Can you work these out from the model? Positions are in its coordinate system, mm. A direction names the side the tool comes from. Round coordinates to 2 decimals unless told otherwise and drop trailing zeros. Order: outer loops, then holes, each group sorted by start corner. A loop starts at its lowest first (then second) coordinate and runs counter-clockwise, first axis right, second up.
Q1. If we section it at B-B (y = 37): Please give me the cut outline in (x, z), plus the area to 3 significant figures.
Q2. We'd pull the mould along Z, two halves only. Please class faces 1 (the face through (7, 0, -5)), 2 (the face through (6.8, 22.5, -4.7)), 3 (the face through (6.84, 44.4, -10.93)), 4 (the face through (7, 23, 0)): pulls with the +Z half, pulls with the -Z half, needs draft (parallel to the pull), parting line crosses it, or undercut.
Q3. For faces 5 (the face through (7, 45, -5)), 6 (the face through (7, 33, -8.681)), which set-ups out of +Z, -Z, +X, -X, +Y, -Y let a thin tool reach every point of the face, with its end or its side?
Q4. If we section it at C-C (z = -5.5): Please give me the cut outline in (x, y).
Q5. If we section it at A-A (z = -7.5): Please give me the cut outline in (x, y).
Q6. If I drill on line 1 (Z direction, x = 5.25, y = 43); line 2 (Y direction, x = 5.25, z = -6.5); line 3 (Y direction, x = 8.5, z = -5.5), over which ranges is the centre line in solid material (lowest first)?
Q7. If we section it at D-D (x = 7.25): Please give me the cut outline in (y, z).
Autodesk Inventor part; units mm, degrees
ref_plane "YZ Plane" through (0, 0, 0) normal (1, 0, 0) x (0, 1, 0)
ref_plane "XZ Plane" through (0, 0, 0) normal (0, 1, 0) x (-1, 0, 0)
ref_plane "XY Plane" through (0, 0, 0) normal (0, 0, 1) x (1, 0, 0)
sketch "スケッチ1" plane through (0, 0, 0) normal (1, 0, 0) x (0, 1, 0)
  line L0 (45, 0) -> (0, 0)
  line L1 (0, 0) -> (0, -11.5)
  line L2 (0, -11.5) -> (45, -11.5)
  line L3 (45, -11.5) -> (45, 0)
  dimension "d0" = 45
  dimension "d1" = 11.5
extrude "押し出し1" add sketch "スケッチ1" along normal blind 13.5
sketch "スケッチ2" plane through (13.5, 0, 0) normal (1, 0, 0) x (0, 0, -1)
  circle A0 centre (1.5, 43) radius 0.8
  circle A1 centre (9.4807, 43) radius 0.8
  circle A2 centre (9.5, 2) radius 0.8
  circle A3 centre (1.5, 2) radius 0.8
  circle A4 centre (5.5, 22.5) radius 0.8
  point P0 (0, 0)
extrude "押し出し2" cut sketch "スケッチ2" against normal through all
fillet "フィレット1" radius 2 2 edges at (6.75, 45, -11.5) (6.75, 0, -11.5)
sketch "スケッチ4" plane through (13.5, 0, 0) normal (1, 0, 0) x (0, 0, -1)
  line L0 (2.3, 40) -> (8.6807, 40)
  line L1 (8.6807, 40) -> (8.6807, 25.5)
  line L2 (8.6807, 25.5) -> (2.3, 25.5)
  line L3 (2.3, 25.5) -> (2.3, 40)
  line L4 (2.3, 19.5) -> (8.6807, 19.5)
  line L5 (8.6807, 19.5) -> (8.6807, 5)
  line L6 (8.6807, 5) -> (2.3, 5)
  line L7 (2.3, 5) -> (2.3, 19.5)
  circle A0 centre (1.5, 43) radius 0.8
  arc A1 (9.5, 0) -> (11.5, 2) centre (9.5, 2) ccw
  line L8 (11.5, 2) -> (11.5, 43)
  arc A2 (11.5, 43) -> (9.5, 45) centre (9.5, 43) ccw
  line L9 (9.5, 45) -> (0, 45)
  line L10 (0, 45) -> (0, 0)
  line L11 (0, 0) -> (9.5, 0)
  circle A3 centre (5.5, 22.5) radius 0.8
  circle A4 centre (9.5, 2) radius 0.8
  circle A5 centre (1.5, 2) radius 0.8
  circle A6 centre (9.4807, 43) radius 0.8
  circle A7 centre (1.5, 43) radius 0.8
  dimension "d9" = 3
  dimension "d10" = 3
  dimension "d11" = 3
  dimension "d12" = 3
extrude "押し出し3" cut sketch "スケッチ4" against normal through all contours L0 L1 L2 L3 | L4 L5 L6 L7
properties part number "chest_cover_stopper"
Solution:
1. outline: (0, -11.5) - (13.5, -11.5) - (13.5, -8.68) - (0, -8.68) - close; (0, -2.3) - (13.5, -2.3) - (13.5, 0) - (0, 0) - close
1. area: 69.1 mm2
2. face 1: needs draft
2. face 2: undercut
2. face 3: pulls with the -Z half
2. face 4: pulls with the +Z half
3. face 5: +Z, -Z, +X, -X, +Y
3. face 6: +X, -X
4. outline: (0, 0) - (13.5, 0) - (13.5, 5) - (0, 5) - close; (0, 19.5) - (13.5, 19.5) - (13.5, 21.7) - (0, 21.7) - close; (0, 23.3) - (13.5, 23.3) - (13.5, 25.5) - (0, 25.5) - close; (0, 40) - (13.5, 40) - (13.5, 45) - (0, 45) - close
5. outline: (0, 0) - (13.5, 0) - (13.5, 5) - (0, 5) - close; (0, 19.5) - (13.5, 19.5) - (13.5, 25.5) - (0, 25.5) - close; (0, 40) - (13.5, 40) - (13.5, 45) - (0, 45) - close
6. line 1: z = -11.5 to -10.28, -8.68 to -2.3, -0.7 to 0
6. line 2: y = 0 to 5, 19.5 to 25.5, 40 to 45
6. line 3: y = 0 to 5, 19.5 to 21.7, 23.3 to 25.5, 40 to 45
7. outline: (0, -9.5) arc R2 ccw to (2, -11.5) - (43, -11.5) arc R2 ccw to (45, -9.5) - (45, 0) - (0, 0) - close; hole circle Ø1.6 at (2, -9.5); hole circle Ø1.6 at (2, -1.5); hole (5, -8.68) - (19.5, -8.68) - (19.5, -2.3) - (5, -2.3) - close; hole circle Ø1.6 at (22.5, -5.5); hole (25.5, -8.68) - (40, -8.68) - (40, -2.3) - (25.5, -2.3) - close; hole circle Ø1.6 at (43, -9.48); hole circle Ø1.6 at (43, -1.5)
